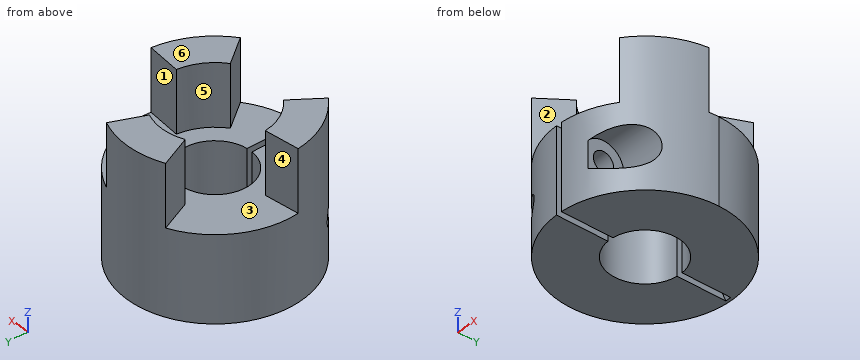
Autodesk Inventor part; units mm, degrees
ref_plane "Work Plane1" through (14.9, 0, 0) normal (1, 0, 0) x (0, 1, 0)
ref_plane "XZ Plane" through (0, 0, 0) normal (0, 1, 0) x (-1, 0, 0)
ref_plane "XY Plane" through (0, 0, 0) normal (0, 0, 1) x (1, 0, 0)
sketch "Sketch1" plane through (0, 0, 0) normal (0, 0, 1) x (1, 0, 0)
  circle A0 centre (0, 0) radius 14.89
  circle A1 centre (0, 0) radius 6
  circle A2 centre (0, 0) radius 3.175
  dimension "d0" = 29.78
  dimension "d1" = 12
  dimension "d41" = 6.35
extrude "Extrusion1" add sketch "Sketch1" along normal blind 25 contours A0
sketch "Sketch2" plane through (0, 0, 25) normal (0, 0, 1) x (1, 0, 0)
  circle A0 centre (0, 0) radius 14.89
  circle A1 centre (0, 0) radius 9
  circle A2 centre (0, 0) radius 14.89
  line L0 (-3.6007, 8.2483) -> (-5.9571, 13.6464)
  line L1 (5.9571, 13.6464) -> (3.6007, 8.2483)
  line L2 (-5.3429, -7.2425) -> (-8.8396, -11.9822)
  line L3 (-14.7967, -1.6642) -> (-8.9436, -1.0059)
  line L4 (8.9436, -1.0059) -> (14.7967, -1.6642)
  line L5 (8.8396, -11.9822) -> (5.3429, -7.2425)
  dimension "d14" = 18
  dimension "d24" = 360
extrude "Extrusion2" cut sketch "Sketch2" against normal blind 10.5 contours A0 L4 A1 L1 | L0 A1 L3 A0 | A1 | A0 L2 A1 L5
ref_plane "Work Plane1" through (14.9, 0, 0) normal (1, 0, 0) x (0, 1, 0)
sketch "Sketch3" plane through (14.9, 0, 0) normal (1, 0, 0) x (0, 1, 0)
  line L0 (-1.6642, 14.5) -> (-1.6642, 25)
  line L1 (-11.9822, 25) -> (-1.6642, 25)
  line L2 (-11.9822, 25) -> (-11.9822, 14.5)
  line L3 (-11.9822, 14.5) -> (-11.9822, 14.5)
  line L4 (-11.9822, 14.5) -> (-11.9822, 25)
  line L5 (-1.6642, 25) -> (-11.9822, 25)
  line L6 (-1.6642, 25) -> (-1.6642, 14.5)
  line L7 (-1.6642, 14.5) -> (13.6464, 14.5)
  line L8 (13.6464, 14.5) -> (13.6464, 25)
  line L9 (13.6464, 25) -> (13.6464, 25)
  line L10 (13.6464, 25) -> (13.6464, 14.5)
  line L11 (13.6464, 14.5) -> (-1.6642, 14.5)
  line L12 (14.89, 0) -> (-14.89, 0)
  line L13 (14.89, 25) -> (13.6464, 25)
  line L14 (14.89, 25) -> (14.89, 0)
  line L15 (14.89, 0) -> (14.89, 25)
  line L16 (-14.89, 0) -> (-14.89, 14.5)
  line L17 (14.89, 0) -> (-14.89, 0)
  line L18 (-14.89, 14.5) -> (-14.89, 0)
  line L19 (-7.89, 0) -> (-14.89, 0)
  line L20 (-14.89, 0) -> (-14.89, 14.5)
  line L21 (-14.89, 7.25) -> (-7.89, 7.25)
  circle A0 centre (-11.39, 7.25) radius 3.5
  circle A1 centre (-11.39, 7.25) radius 1.75
  point P0 (0, 0)
  dimension "d27" = 29.78
  dimension "d30" = 3.5
extrude "Extrusion3" cut sketch "Sketch3" against normal blind 10
extrude "Extrusion4" cut sketch "Sketch3" against normal blind 30 contours A1 L21 | L21 A1
sketch "Sketch4" plane through (0, 0, 0) normal (0, 0, -1) x (-1, 0, 0)
  arc A0 (-8.8396, -11.9822) -> (8.8396, -11.9822) centre (0, 0) ccw
  line L0 (0, 0) -> (-0.5, 0)
  line L1 (-0.5, 0) -> (-0.5, -14.8816)
  line L2 (0, 0) -> (0.5, 0)
  line L3 (0.5, 0) -> (0.5, -14.8816)
  line L4 (-0.5, 0) -> (-0.5, 14.8816)
  line L5 (0.5, 0) -> (0.5, 14.8816)
  arc A1 (5.3429, -7.2425) -> (8.9436, -1.0059) centre (0, 0) ccw
  circle A2 centre (0, 0) radius 14.89
  point P0 (-8.8396, 11.9822)
  dimension "d33" = 0.5
  dimension "d34" = 0.5
extrude "Extrusion5" cut sketch "Sketch4" against normal blind 15 contours L1 L0 L2 L3 A0
sketch "Sketch5" plane through (-0.5, -14.8816, 0) normal (1, 0, 0) x (0, 0, -1)
  line L0 (0, 0) -> (-14.5, 0)
  line L1 (-14.5, 0) -> (-14.5, 2.8994)
  line L2 (-14.5, 2.8994) -> (-25, 2.8994)
  line L3 (-25, 13.2174) -> (-25, 2.8994)
  line L4 (-25, 13.2174) -> (-14.5, 13.2174)
  line L5 (-14.5, 13.2174) -> (-14.5, 28.528)
  line L6 (-14.5, 28.528) -> (-25, 28.528)
  line L7 (-25, 28.528) -> (-25, 28.528)
  line L8 (-25, 28.528) -> (-14.5, 28.528)
  line L9 (-14.5, 28.528) -> (-14.5, 13.2174)
  line L10 (-14.5, 13.2174) -> (-25, 13.2174)
  line L11 (-25, 2.8994) -> (-25, 13.2174)
  line L12 (-25, 2.8994) -> (-14.5, 2.8994)
  line L13 (-14.5, 2.8994) -> (-14.5, 0)
  line L14 (-14.5, 0) -> (0, 0)
  line L15 (0, 0) -> (0, 0)
  line L16 (-4.9878, 0.8209) -> (-9.5122, 0.8209)
  line L17 (-14.5, 8.9025) -> (0, 8.9025)
  line L18 (0, 8.9025) -> (0, 8.9025)
  line L19 (0, 8.9025) -> (-14.5, 8.9025)
  line L20 (-14.5, 8.9025) -> (-14.5, 8.9025)
  line L21 (-14.5, 20.8816) -> (-14.5, 8.9025)
  line L22 (-14.5, 20.8816) -> (0, 20.8816)
  line L23 (0, 29.7716) -> (0, 0)
  line L24 (-14.5, 20.8816) -> (-14, 20.8816)
  line L25 (0, 29.7716) -> (0, 29.2716)
  line L26 (0, 29.2716) -> (-14, 20.8816)
  line L27 (-14.5, 20.8585) -> (0, 20.8585)
  line L28 (0, 8.9025) -> (0, 20.8816)
  line L29 (-14, 20.8816) -> (-14.0385, 20.8585)
  line L30 (-14.5, 18.0566) -> (0, 18.0566)
  line L31 (-14.5, 18.0566) -> (-14.5, 11.7462)
  line L32 (-14.5, 18.0145) -> (0, 18.0145)
  line L33 (-14.5, 18.0145) -> (-14, 18.0145)
  line L34 (-14, 18.0145) -> (0, 29.2716)
  point P0 (0, 14.8816)
  point P1 (-7.25, 1.7416)
  point P2 (-13.9476, 18.0566)
  dimension "d37" = 0.5
  dimension "d38" = 0.5
  dimension "d42" = 0.5
extrude "Extrusion6" cut sketch "Sketch5" along normal blind 1 contours L32 L34 L30 L23 | L30 L34 L27 L23 | L32 L5 L30 L34 | L27 L34 L22 L23 | L30 L5 L27 L34 | L22 L34 L23 | L27 L29 L22 L34 | L22 L26 L34
properties part number "PHAN NHOM"
Source: CAD feature listing. Evaluate the final solid. Frame: model axes, mm. Face numbers are marked on the shaded views. A direction names the side the tool comes from. Round coordinates to 2 decimals unless told otherwise and drop trailing zeros. Loops run counter-clockwise (first coordinate to the right, second up) from the corner with the lowest first, then second, coordinate; pieces in that order, holes last.
1. Mould query, pull axis X, two halves, no side actions, for the marked faces 4, 5 and 6. Classes: released by +X, released by -X, zero draft, split by the parting line, or undercut.
2. Access query for the marked faces 1, 2 and 3. Directions: +Z, -Z, +X, -X, +Y, -Y. A direction counts if a zero-diameter tool reaches every point of the face in a straight line with its end or side. Return the directions, or none.
3. Section query B-B on z = 21.75. Output: boundary loops of the cut face in (x, y).
4. Section query D-D on x = 12. Output: boundary loops of the cut face in (y, z).
5. Section query A-A on x = 1.75. Output: boundary loops of the cut face in (y, z).
6. Contact query for flat-ended pins moving along their axis: pin 1 (2 mm diameter, centred on y = 8.5, z = 9, fed in from +X); pin 2 (4 mm diameter, centred on y = -11.39, z = 7.25, fed in from -X); pin 3 (4 mm diameter, centred on y = -11.39, z = 7.25, fed in from +X). Output: stop coordinate, or through.
7. Ray query, L1, parallel to Z at x = 3.05, y = -11.39; L2, parallel to X at y = 0, z = 10.75; L3, parallel to Z at x = -2.25, y = -8.75. Return the intervals inside material, ascending.
8. Section query C-C on y = -11.39. Output: boundary loops of the cut face in (x, z), and give its area (3 significant figures).
Answers below:
1. face 4: released by -X
1. face 5: undercut
1. face 6: zero draft
2. face 1: +Z, +X, +Y
2. face 2: +Z, -Y
2. face 3: +Z
3. outline: (-14.8, -1.66) arc R14.89 ccw to (-8.84, -11.98) - (-5.34, -7.24) arc R9 cw to (-8.94, -1.01) - close; (-5.96, 13.65) - (-3.6, 8.25) arc R9 cw to (3.6, 8.25) - (5.96, 13.65) arc R14.89 ccw to start; (5.34, -7.24) - (8.84, -11.98) arc R14.89 ccw to (14.8, -1.66) - (8.94, -1.01) arc R9 cw to start
4. outline: (-8.82, 0) - (8.82, 0) - (8.82, 14.5) - (-1.35, 14.5) - (-1.35, 25) - (-8.82, 25) - (-8.82, 9.62) arc R3.5 cw to (-8.82, 4.88) - close
5. outline: (-14.79, 0) - (-5.74, 0) - (-5.74, 14.5) - (-14.79, 14.5) - close; (5.74, 0) - (14.79, 0) - (14.79, 25) - (8.83, 25) - (8.83, 14.5) - (5.74, 14.5) - close; hole circle Ø3.5 at (-11.39, 7.25)
6. pin 1: stops at x = 12.86
6. pin 2: stops at x = -11.56
6. pin 3: stops at x = 4.9
7. L1: z = 0 to 5.5, 9 to 14.5
7. L2: x = -14.89 to -6, 6 to 14.89
7. L3: z = 0 to 14.5
8. outline: (-9.59, 0) - (-0.5, 0) - (-0.5, 5.5) - (-9.59, 5.5) - close; (-9.59, 9) - (-0.5, 9) - (-0.5, 14.5) - (-8.4, 14.5) - (-8.4, 25) - (-9.59, 25) - close; (0.5, 0) - (9.59, 0) - (9.59, 3.75) - (4.9, 3.75) - (4.9, 5.5) - (0.5, 5.5) - close; (0.5, 9) - (4.9, 9) - (4.9, 10.75) - (9.59, 10.75) - (9.59, 25) - (8.4, 25) - (8.4, 14.5) - (0.5, 14.5) - close
8. area: 209 mm2
